Geometry: see drawing. Coordinates: mm, zero at the bounding-box minimum. A direction names the side the tool comes from. Coordinates: 2 decimals unless noted, no trailing zeros. Loops run counter-clockwise (first coordinate to the right, second up) from the corner with the lowest first, then second, coordinate; pieces in that order, holes last. Notation, with made-up numbers: (19, 21.25) -> (41, 21.25) arc R32 ccw to (41, 56.25) -> close; hole circle Ø8 at (-16.75, 67). An arc over 180 degrees is marked (long way). Answer as a JSON object with one key per item and string values.
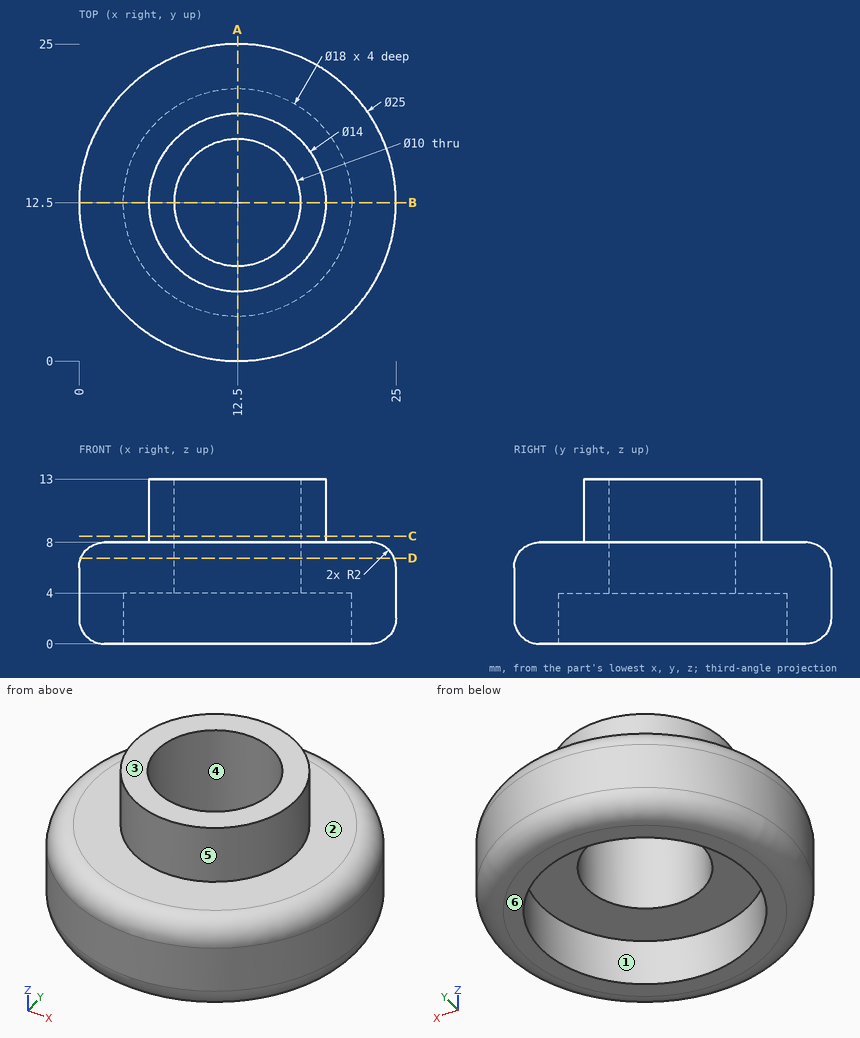
1. Line query: line 1 along Y through (x, z) = (12.5, 2.1); line 2 along Y through (x, z) = (12.5, 6); line 3 along Z through (x, y) = (16.25, 17.5). Output: solid intervals per line, ascending.
Reply:
{"line 1": "y = 0 to 3.5, 21.5 to 25", "line 2": "y = 0 to 7.5, 17.5 to 25", "line 3": "z = 4 to 13"}
2. Pin query (flat end, axial travel): P1, Ø5, axis at x = 14, y = 15, coming from the +Z side; P2, Ø1.5, axis at x = 19.5, y = 9, coming from the -Z side; P3, Ø6, axis at x = 4.5, z = 3, coming from the -Y side. Return the tip coordinate at first contact, or that it passes through.
Reply:
{"P1": "stops at z = 13", "P2": "stops at z = 4", "P3": "stops at y = 1.04"}
3. Section query C-C (z = 8.5). Return loops of the section in (x, y), plus the area to 3 significant figures.
Reply:
{"outline": "circle Ø14 at (12.5, 12.5); hole circle Ø10 at (12.5, 12.5)", "area": "75.4 mm2"}
4. Mould query, pull axis Y, two halves, no side actions, for the marked faces 4, 5 and 6. Classes: pulls with the +Y half, pulls with the -Y half, needs draft (parallel to the pull), parting line crosses it, or undercut.
Reply:
{"face 4": "undercut", "face 5": "parting line crosses it", "face 6": "needs draft"}
5. Section query D-D (z = 6.75). Return loops of the section in (x, y).
Reply:
{"outline": "circle Ø24.71 at (12.5, 12.5); hole circle Ø10 at (12.5, 12.5)"}
6. Access query for the marked faces 1, 2 and 3. Directions: +Z, -Z, +X, -X, +Y, -Y. A direction counts if a zero-diameter tool reaches every point of the face in a straight line with its end or side. Return the directions, or none.
Reply:
{"face 1": "-Z", "face 2": "+Z", "face 3": "+Z, +X, -X, +Y, -Y"}
7. Section query A-A (x = 12.5). Return loops of the section in (y, z).
Reply:
{"outline": "(0, 2) arc R2 ccw to (2, 0) -> (3.5, 0) -> (3.5, 4) -> (7.5, 4) -> (7.5, 13) -> (5.5, 13) -> (5.5, 8) -> (2, 8) arc R2 ccw to (0, 6) -> close; (17.5, 4) -> (21.5, 4) -> (21.5, 0) -> (23, 0) arc R2 ccw to (25, 2) -> (25, 6) arc R2 ccw to (23, 8) -> (19.5, 8) -> (19.5, 13) -> (17.5, 13) -> close"}
